Geometry check sheet. Reference: the model listing, model coordinates, mm. A direction names the side the tool comes from. Coordinates: 2 decimals unless noted, no trailing zeros. Write each loop counter-clockwise with the first axis right and the second up, starting at its lowest first coordinate (ties: lowest second). Pieces come first, ordered by that corner, then holes. Notation, with made-up numbers: (69.25, 56.5) -> (104.25, 56.5) arc R15 cw to (104.25, 61.5) -> close; hole circle Ø10 at (9, 72.25). An arc over 180 degrees is marked (long way). Answer as CSV lines item,"result".
```python
from build123d import *

# Parameters (mm, degrees)
SKETCH1_R                 = 4
BOSS_EXTRUDE1_DEPTH       = 6.35
F_5_0MM_DOWEL_SLOT1_DEPTH = 6.35
SKETCH5_R                 = 5.25
CUT_EXTRUDE1_DEPTH        = 3


# Read off the part's stored shape, not the designer's step: Ø5.0mm Dowel Slot1
with BuildPart() as part:
    # Sketch1 → Boss-Extrude1 (new body)
    with BuildSketch(Plane.XY):
        with BuildLine():
            Line((-27.999999098, 10), (48.000000902, 10))
            ThreePointArc((48.000000902, 10), (49.414214465, 9.414213562), (50.000000902, 8))
            Line((50.000000902, 8), (50.000000902, -30))
            ThreePointArc((50.000000902, -30), (48.535534808, -33.535533906), (45.000000902, -35))
            Line((45.000000902, -35), (-24.999999098, -35))
            ThreePointArc((-24.999999098, -35), (-28.535533003, -33.535533906), (-29.999999098, -30))
            Line((-29.999999098, -30), (-29.999999098, 8))
            ThreePointArc((-29.999999098, 8), (-29.41421266, 9.414213562), (-27.999999098, 10))
        make_face()
        with Locations((10.000000902, -20.95)):
            Circle(SKETCH1_R, mode=Mode.SUBTRACT)
    extrude(amount=BOSS_EXTRUDE1_DEPTH)

    # Ø5.0mm Dowel Slot1 outline → Ø5.0mm Dowel Slot1 (cut)
    with BuildSketch(Plane.XY):
        with BuildLine():
            Line((22.500000902, -3.85), (22.500000902, 3.85))
            ThreePointArc((22.500000902, 3.85), (20.000000902, 6.35), (17.500000902, 3.85))
            Line((17.500000902, 3.85), (17.500000902, -3.85))
            ThreePointArc((17.500000902, -3.85), (20.000000902, -6.35), (22.500000902, -3.85))
        make_face()
        with BuildLine():
            Line((-17.499999098, -3.85), (-17.499999098, 3.85))
            ThreePointArc((-17.499999098, 3.85), (-19.999999098, 6.35), (-22.499999098, 3.85))
            Line((-22.499999098, 3.85), (-22.499999098, -3.85))
            ThreePointArc((-22.499999098, -3.85), (-19.999999098, -6.35), (-17.499999098, -3.85))
        make_face()
        with BuildLine():
            Line((2.500000902, -3.85), (2.500000902, 3.85))
            ThreePointArc((2.500000902, 3.85), (9.02e-07, 6.35), (-2.499999098, 3.85))
            Line((-2.499999098, 3.85), (-2.499999098, -3.85))
            ThreePointArc((-2.499999098, -3.85), (9.02e-07, -6.35), (2.500000902, -3.85))
        make_face()
        with BuildLine():
            Line((42.500000902, -3.85), (42.500000902, 3.85))
            ThreePointArc((42.500000902, 3.85), (40.000000902, 6.35), (37.500000902, 3.85))
            Line((37.500000902, 3.85), (37.500000902, -3.85))
            ThreePointArc((37.500000902, -3.85), (40.000000902, -6.35), (42.500000902, -3.85))
        make_face()
    extrude(amount=F_5_0MM_DOWEL_SLOT1_DEPTH, mode=Mode.SUBTRACT)

    # Sketch5 → Cut-Extrude1 (cut)
    with BuildSketch(Plane(origin=(0, 0, 0), x_dir=(-1, 0, 0), z_dir=(0, 0, -1))):
        with Locations((-10.000000902, -20.95)):
            Circle(SKETCH5_R)
    extrude(amount=-CUT_EXTRUDE1_DEPTH, mode=Mode.SUBTRACT)


solid = part.part
```
Item 1: Cross-section at D-D, the plane y = -20.95. Record the cut outline in (x, z).
Responses:
outline,"(-30, 0) -> (4.75, 0) -> (4.75, 3) -> (6, 3) -> (6, 6.35) -> (-30, 6.35) -> close; (14, 3) -> (15.25, 3) -> (15.25, 0) -> (50, 0) -> (50, 6.35) -> (14, 6.35) -> close"
Item 2: Depth check by flat-ended pin: pin 1 Ø3 at (x, y) = (8, -23.5) entering from -Z. Enter the tip coordinate at first touch or a pass-through.
Responses:
pin 1,"stops at z = 3"
Item 3: Cross-section at C-C, the plane y = 1.5. Record the cut outline in (x, z).
Responses:
outline,"(-30, 0) -> (-22.5, 0) -> (-22.5, 6.35) -> (-30, 6.35) -> close; (-17.5, 0) -> (-2.5, 0) -> (-2.5, 6.35) -> (-17.5, 6.35) -> close; (2.5, 0) -> (17.5, 0) -> (17.5, 6.35) -> (2.5, 6.35) -> close; (22.5, 0) -> (37.5, 0) -> (37.5, 6.35) -> (22.5, 6.35) -> close; (42.5, 0) -> (50, 0) -> (50, 6.35) -> (42.5, 6.35) -> close"
Item 4: Set-up check for faces 1 (the flat face through (-30, -11, 3)), 2 (the cylindrical face through (4.992, -19.373, 1.479)), 3 (the cylindrical face through (-19.95, 6.35, 3.13)): record each of +Z, -Z, +X, -X, +Y, -Y from which the full face is reachable in a straight line by a thin tool's end or side.
Responses:
face 1,"+Z, -Z, -X, +Y, -Y"
face 2,"-Z"
face 3,"+Z, -Z"
Item 5: Cross-section at A-A, the plane x = 10. Record the cut outline in (y, z), plus the area to 3 significant figures.
Responses:
outline,"(-35, 0) -> (-26.2, 0) -> (-26.2, 3) -> (-24.95, 3) -> (-24.95, 6.35) -> (-35, 6.35) -> close; (-16.95, 3) -> (-15.7, 3) -> (-15.7, 0) -> (10, 0) -> (10, 6.35) -> (-16.95, 6.35) -> close"
area,"227 mm2"
Item 6: Thickness scan on probe 1 along X at (y, z) = (-3.5, 4.5); probe 2 along Y at (x, z) = (10, 4); probe 3 along Y at (x, z) = (0, 6.25). Record the ranges inside material, lowest first.
Responses:
probe 1,"x = -30 to -22.5, -17.5 to -2.5, 2.5 to 17.5, 22.5 to 37.5, 42.5 to 50"
probe 2,"y = -35 to -24.95, -16.95 to 10"
probe 3,"y = -35 to -6.35, 6.35 to 10"
Item 7: Release check for a two-part mould opening along Y. For faces 4 (the flat face through (10, -35, 3)), 5 (the flat face through (9, 10, 3)), 6 (the flat face through (11, -12, 0)), 7 (the cylindrical face through (40.05, 6.35, 3.13)) record: +Y half, -Y half, draft (parallel to the pull), parting line (faces both ways), or undercut.
Responses:
face 4,"-Y half"
face 5,"+Y half"
face 6,"draft"
face 7,"undercut"
Item 8: Cross-section at B-B, the plane z = 4. Record the cut outline in (x, y), plus the area to 3 significant figures.
Responses:
outline,"(-30, -30) arc R5 ccw to (-25, -35) -> (45, -35) arc R5 ccw to (50, -30) -> (50, 8) arc R2 ccw to (48, 10) -> (-28, 10) arc R2 ccw to (-30, 8) -> close; hole (-22.5, -3.85) arc R2.5 ccw to (-17.5, -3.85) -> (-17.5, 3.85) arc R2.5 ccw to (-22.5, 3.85) -> close; hole (-2.5, -3.85) arc R2.5 ccw to (2.5, -3.85) -> (2.5, 3.85) arc R2.5 ccw to (-2.5, 3.85) -> close; hole circle Ø8 at (10, -20.95); hole (17.5, -3.85) arc R2.5 ccw to (22.5, -3.85) -> (22.5, 3.85) arc R2.5 ccw to (17.5, 3.85) -> close; hole (37.5, -3.85) arc R2.5 ccw to (42.5, -3.85) -> (42.5, 3.85) arc R2.5 ccw to (37.5, 3.85) -> close"
area,"3,300 mm2"
